from build123d import *

# Parameters (mm, degrees)
BOSS_EXTRUDE1_DEPTH     = 133
SKETCH3_W               = 20
SKETCH3_H               = 20
CUT_EXTRUDE1_DEPTH      = 1040.5
CUT_EXTRUDE2_DEPTH      = 138.347005792
CUT_EXTRUDE2_DEPTH_BACK = 138.347005792
CUT_EXTRUDE3_DEPTH      = 138.347005792
CUT_EXTRUDE3_DEPTH_BACK = 138.347005792


with BuildPart() as part:
    # Sketch1 → Boss-Extrude1 (new body)
    with BuildSketch(Plane(origin=(0, 0, 0), x_dir=(1, 0, 0), z_dir=(0, 1, 0))):
        with BuildLine():
            Line((2.8, 0), (22.8, 0))
            ThreePointArc((22.8, 0), (24.779898987, -0.820101013), (25.6, -2.8))
            Line((25.6, -2.8), (25.6, -22.8))
            ThreePointArc((25.6, -22.8), (24.779898987, -24.779898987), (22.8, -25.6))
            Line((22.8, -25.6), (2.8, -25.6))
            ThreePointArc((2.8, -25.6), (0.820101013, -24.779898987), (0, -22.8))
            Line((0, -22.8), (0, -2.8))
            ThreePointArc((0, -2.8), (0.820101013, -0.820101013), (2.8, 0))
        make_face()
    extrude(amount=BOSS_EXTRUDE1_DEPTH)

    # Sketch3 → Cut-Extrude1 (cut)
    with BuildSketch(Plane(origin=(0, 0, 0), x_dir=(-1, 0, 0), z_dir=(0, -1, 0))):
        with Locations((-12.8, -12.8)):
            Rectangle(SKETCH3_W, SKETCH3_H)
    extrude(amount=-CUT_EXTRUDE1_DEPTH, mode=Mode.SUBTRACT)

    # Sketch4 → Cut-Extrude2 (cut, two sides: drawn at the far end of the back side and taken through both)
    with BuildSketch(Plane(origin=(0, 0, 22.8), x_dir=(-1, 0, 0), z_dir=(0, 0, -1)).offset(-CUT_EXTRUDE2_DEPTH_BACK)):
        Polygon((-280.166183006, 251.706160643), (-25.6, 133), (0, 121.062523951), (254.566183006, 2.356363308), (491.978504292, 511.48872932), (-42.75386172, 760.838526655), align=None)
    extrude(amount=CUT_EXTRUDE2_DEPTH + CUT_EXTRUDE2_DEPTH_BACK, mode=Mode.SUBTRACT)

    # Sketch5 → Cut-Extrude3 (cut, two sides: drawn at the far end of the back side and taken through both)
    with BuildSketch(Plane(origin=(0, 0, 22.8), x_dir=(-1, 0, 0), z_dir=(0, 0, -1)).offset(-CUT_EXTRUDE3_DEPTH_BACK)):
        Polygon((243.251558225, -140.441352622), (0, 0), (-25.6, 14.780166891), (-268.851558225, 155.221519513), (-549.734263468, -331.281596936), (-37.631147019, -626.944469071), align=None)
    extrude(amount=CUT_EXTRUDE3_DEPTH + CUT_EXTRUDE3_DEPTH_BACK, mode=Mode.SUBTRACT)


solid = part.part
The listing builds one solid part. Answer for the finished solid, in the listing's coordinates (mm). A direction names the side the tool comes from. Give positions to 0.01 mm unless a question says otherwise; leave off trailing zeros. Loops run counter-clockwise (first coordinate to the right, second up) from the corner with the lowest first, then second, coordinate; pieces in that order, holes last. Notation, with made-up numbers: M 72,-2.5 L 121,-2.5 A31 cw 121,36.5 Z; hole C -1.5,-14 d6. An arc over 180 degrees is marked long. Answer as CSV lines item,"result".
Item 1: The part is cut by section B-B (y = 53). Give the vertices of the cut face in (x, z).
Values follow:
outline,"M 0,2.8 A2.8 ccw 2.8,0 L 22.8,0 A2.8 ccw 25.6,2.8 L 25.6,22.8 A2.8 ccw 22.8,25.6 L 2.8,25.6 A2.8 ccw 0,22.8 Z; hole M 2.8,2.8 L 22.8,2.8 L 22.8,22.8 L 2.8,22.8 Z"
Item 2: Straight lines are drawn through the part: line 1 along X through (y, z) = (74, 8.25); line 2 along Z through (x, y) = (24.25, 116). For each, find the intervals that lie inside material, in ascending order. Write a range as [from, to].
Values follow:
line 1,"x = [0, 2.8], [22.8, 25.6]"
line 2,"z = [0.4, 25.2]"
Item 3: The mould has two halves that part along Z. Classify faces 1 (the flat face through (12.621, 7.287, 24.357)), 2 (the cylindrical face through (24.8, 72.24, 24.76)), 3 (the flat face through (13, 66, 2.8)): released by +Z, released by -Z, zero draft, split by the parting line, or undercut.
Values follow:
face 1,"zero draft"
face 2,"released by +Z"
face 3,"undercut"
Item 4: Given pin 1 Ø2 at (x, z) = (11.5, 22.5) entering from -Y; pin 2 Ø10 at (x, z) = (5, 16.5) entering from +Y; pin 3 Ø10 at (x, z) = (11.5, 4.5) entering from +Y, each flat-ended and moving along its own axis, determine where each tip first touches the part or whether it passes through.
Values follow:
pin 1,"stops at y = 6.09"
pin 2,"stops at y = 122.37"
pin 3,"stops at y = 128.62"
Item 5: Which of the six approach directions +Z, -Z, +X, -X, +Y, -Y give full straight-line access (tool end or side, diameter ignored) to faces 4 (the flat face through (13, 66, 22.8)), 5 (the cylindrical face through (0.8, 60.33, 0.84))?
Values follow:
face 4,"+Y, -Y"
face 5,"-Z, -X, +Y, -Y"
Item 6: The part is cut by section A-A (z = 20.25). Give the vertices of the cut face in (x, y), and give its area (3 significant figures).
Values follow:
outline,"M 0,0 L 2.8,1.62 L 2.8,122.37 L 0,121.06 Z; M 22.8,13.16 L 25.6,14.78 L 25.6,133 L 22.8,131.69 Z"
area,"670 mm^2"
Item 7: The part is cut by section C-C (x = 10). Give the vertices of the cut face in (y, z), and give its area (3 significant figures).
Values follow:
outline,"M 5.77,0 L 125.73,0 L 125.73,2.8 L 5.77,2.8 Z; M 5.77,22.8 L 125.73,22.8 L 125.73,25.6 L 5.77,25.6 Z"
area,"672 mm^2"
